For this review, take the finished solid that the model builds, in its own axes (mm). Give positions to 0.01 mm unless a question says otherwise; leave off trailing zeros. Order: outer loops, then holes, each group sorted by start corner. A loop starts at its lowest first (then second) coordinate and runs counter-clockwise, first axis right, second up. Notation, with made-up numbers: (28.25, 78.5) - (85.25, 78.5) arc R8 cw to (85.25, 88.5) - close; hole circle Ø6 at (19, 4). An arc over 180 degrees is marked (long way). Use a Markdown table: item, result. Add a question column.
1) We need section A-A on y = 70.5. Write out the cut boundary in (x, z), then the cut area to 3 significant figures.
2) Mouldability with a two-part tool opening along Y and no side actions: class faces 1 (the face through (58.52, 41.73, 0.59)), 2 (the face through (77, 67, 0)), 3 (the face through (142.795, 98.181, 0.592)) as released by +Y, released by -Y, zero draft, split by the parting line, or undercut.
3) Wall thickness on L1, parallel to X at y = 72.5, z = 0.3; L2, parallel to Y at x = 68, z = 0.35; L3, parallel to Y at x = 41, z = 1.15: over which ranges is each line inside the solid? List them lowest first.
4) Clearance check with flat-ended pins moving along their axes: P1, Ø0.6, axis at y = 104.5, z = 1, coming from the -X side; P2, Ø3.5, axis at x = 140.26, y = 88.57, coming from the -Z side; P3, Ø0.6, axis at x = 25.5, z = 0.5, coming from the -Y side. State where each tip first meets the part, or that it passes through.
5) We need section B-B on z = 1. Give the number of separate pieces and of enclosed holes in the cut face, then the cut area to 3 significant figures.
6) We need section C-C on x = 35. Write out the cut boundary in (y, z).
7) We need section D-D on x = 70. Write out the cut boundary in (y, z).
```python
from build123d import *

# Parameters (mm, degrees)
ESQUISSE2_R        = 1.6
ESQUISSE2_R_2      = 1.948326961
BOSS_EXTRU_1_DEPTH = 1.2


with BuildPart() as part:
    # Esquisse2 → Boss.-Extru.1 (new body)
    with BuildSketch(Plane.XY):
        Polygon((38.19435, 93.5719), (14.6697, 93.5719), (9.6697, 88.5719), (9.6697, 42.4727), (14.6697, 37.4727), (56.719, 37.4727), (67.2947, 27.9475), (85.586462681, 27.9475), (103.516430018, 23.142256556), (119.601627139, 13.856517967), (132.532309311, 0.926057837), (145.259827189, 13.653794272), (145.259827189, 95.7157), (140.259827189, 100.7157), (95.34435, 100.7157), (95.34435, 103.097), (76.29435, 103.097), (76.29435, 107.859), (57.24435, 107.859), (57.24435, 103.097), (38.19435, 103.097), align=None)
        with Locations((14.6697, 42.4727)):
            Circle(ESQUISSE2_R, mode=Mode.SUBTRACT)
        with Locations((14.6697, 88.5719)):
            Circle(ESQUISSE2_R, mode=Mode.SUBTRACT)
        with Locations((140.259827189, 88.5719)):
            Circle(ESQUISSE2_R, mode=Mode.SUBTRACT)
        with Locations((140.259827189, 42.4727)):
            Circle(ESQUISSE2_R, mode=Mode.SUBTRACT)
        with Locations((56.719, 42.4727)):
            Circle(ESQUISSE2_R_2, mode=Mode.SUBTRACT)
        with BuildLine():
            Line((16.1697, 77.5727), (16.1697, 53.4719))
            ThreePointArc((16.1697, 53.4719), (14.6697, 51.9719), (13.1697, 53.4719))
            Line((13.1697, 53.4719), (13.1697, 77.5727))
            ThreePointArc((13.1697, 77.5727), (14.6697, 79.0727), (16.1697, 77.5727))
        make_face(mode=Mode.SUBTRACT)
        with BuildLine():
            Line((141.759827189, 77.5727), (141.759827189, 53.4719))
            ThreePointArc((141.759827189, 53.4719), (140.259827189, 51.9719), (138.759827189, 53.4719))
            Line((138.759827189, 53.4719), (138.759827189, 77.5727))
            ThreePointArc((138.759827189, 77.5727), (140.259827189, 79.0727), (141.759827189, 77.5727))
        make_face(mode=Mode.SUBTRACT)
    extrude(amount=BOSS_EXTRU_1_DEPTH)


solid = part.part
```
Checked values:
| question | item | result |
|---|---|---|
| 1 | outline | (9.67, 0) - (13.17, 0) - (13.17, 1.2) - (9.67, 1.2) - close; (16.17, 0) - (138.76, 0) - (138.76, 1.2) - (16.17, 1.2) - close; (141.76, 0) - (145.26, 0) - (145.26, 1.2) - (141.76, 1.2) - close |
| 1 | area | 156 mm² |
| 2 | face 1 | undercut |
| 2 | face 2 | zero draft |
| 2 | face 3 | released by +Y |
| 3 | L1 | 9.67 to 13.17, 16.17 to 138.76, 141.76 to 145.26 |
| 3 | L2 | 27.95 to 107.86 |
| 3 | L3 | 37.47 to 103.1 |
| 4 | P1 | x = 57.24 |
| 4 | P2 | z = 0 |
| 4 | P3 | y = 37.47 |
| 5 | separate pieces | 1 |
| 5 | enclosed holes | 7 |
| 5 | area | 9,870 mm² |
| 6 | outline | (37.47, 0) - (93.57, 0) - (93.57, 1.2) - (37.47, 1.2) - close |
| 7 | outline | (27.95, 0) - (107.86, 0) - (107.86, 1.2) - (27.95, 1.2) - close |
